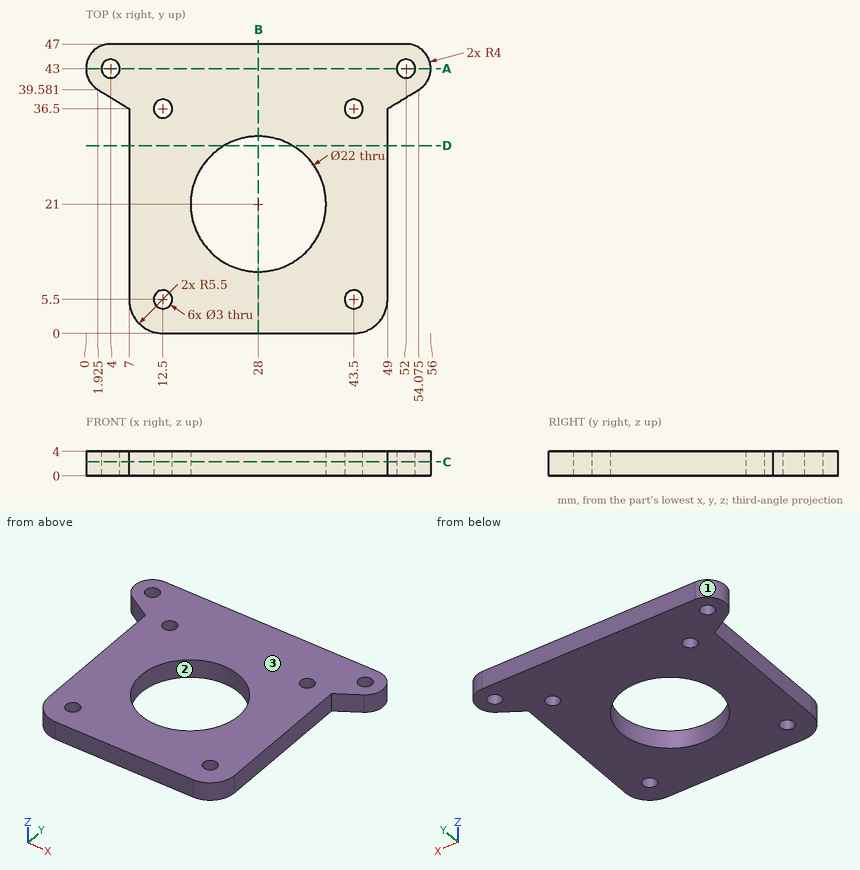
Here's the drawing with two shaded views (mm, measured from the low corner). I have some questions. Coordinates: 2 decimals unless noted, no trailing zeros. Write each loop counter-clockwise with the first axis right and the second up, starting at its lowest first coordinate (ties: lowest second). Pieces come first, ordered by that corner, then holes. Notation, with made-up numbers: M 37.25,82 L 72.25,82 A6 cw 72.25,93 Z; hole C 51.5,67 d6. An arc over 180 degrees is marked long. Write item = value, one per line. Start each with the question number.
Q1. Thinking about a two-plate mould opening in X: for the marked faces 1, 2 and 3, which applies, released by +X, released by -X, zero draft, split by the parting line, or undercut?
Q2. If we section it at C-C, the plane z = 2.3: Write out the boundary of the cut face in (x, y) (1 decimal).
Q3. I'm going to push flat-ended pins straight in: pin 1 (2.5 mm diameter, centred on x = 43.5, y = 36.5, fed in from -Z); pin 2 (1.2 mm diameter, centred on y = 15.5, z = 3, fed in from +X); pin 3 (2 mm diameter, centred on y = 17.5, z = 1.5, fed in from -X). Where does each tip first touch, or does it pass through?
Q4. If we section it at A-A, the plane y = 43: Write out the boundary of the cut face in (x, z).
Q5. If we section it at B-B, the plane x = 28: Write out the boundary of the cut face in (y, z), then the cut area to 3 significant figures.
Q6. If I drill on L1, parallel to Y at x = 43.5, z = 1.5; L2, parallel to Y at x = 28.5, z = 3.2; L3, parallel to Y at x = 43, z = 3.2 (1 decimal), over which ranges is the centre line in solid material (lowest first)? Write a range as [from, to].
Q7. If we section it at D-D, the plane y = 30.5: Write out the boundary of the cut face in (x, z) (1 decimal), then the cut area to 3 significant figures.
Check sheet entries:
q1.face_1 = released by -X
q1.face_2 = undercut
q1.face_3 = zero draft
q2.outline = M 1.9,39.6 L 7,36.5 L 7,5.5 A5.5 ccw 12.5,0 L 43.5,0 A5.5 ccw 49,5.5 L 49,36.5 L 54.1,39.6 A4 ccw 52,47 L 4,47 A4 ccw Z; hole C 4,43 d3; hole C 12.5,5.5 d3; hole C 12.5,36.5 d3; hole C 28,21 d22; hole C 43.5,5.5 d3; hole C 43.5,36.5 d3; hole C 52,43 d3
q3.pin_1 = through
q3.pin_2 = 49
q3.pin_3 = 7
q4.outline = M 0,0 L 2.5,0 L 2.5,4 L 0,4 Z; M 5.5,0 L 50.5,0 L 50.5,4 L 5.5,4 Z; M 53.5,0 L 56,0 L 56,4 L 53.5,4 Z
q5.outline = M 0,0 L 10,0 L 10,4 L 0,4 Z; M 32,0 L 47,0 L 47,4 L 32,4 Z
q5.area = 100 mm²
q6.L1 = [0, 4], [7, 35], [38, 47]
q6.L2 = [0, 10.01], [31.99, 47]
q6.L3 = [0, 4.1], [6.9, 35.1], [37.9, 47]
q7.outline = M 7,0 L 22.5,0 L 22.5,4 L 7,4 Z; M 33.5,0 L 49,0 L 49,4 L 33.5,4 Z
q7.area = 124 mm²
